Could you check a few things on this model? Use its own coordinates, in mm. Give positions to 0.01 mm unless a question says otherwise; leave off trailing zeros. Loops run counter-clockwise (first coordinate to the right, second up) from the corner with the lowest first, then second, coordinate; pieces in that order, holes last. Notation, with made-up numbers: M -27.75,10.25 L -3.75,10.25 A26 cw -3.75,33.25 Z; hole C 61.25,77.5 d2. An arc over 180 degrees is marked long. Use CSV: the item, a comma, the result in double quotes.
```python
from build123d import *

# Parameters (mm, degrees)
SKETCH1_W             = 5
SKETCH1_H             = 112
BOSS_EXTRUDE1_DEPTH   = 5
SKETCH2_W             = 112
SKETCH2_H             = 5
BOSS_EXTRUDE2_DEPTH   = 145
BOSS_EXTRUDE3_DEPTH   = 107
SKETCH5_W             = 150
SKETCH5_H             = 3
CUT_EXTRUDE1_DEPTH    = 30
CHAMFER1_SIZE         = 2
CHAMFER1_SIZE2        = 1.414213562
CHAMFER1_EDGE_2_SIZE  = 2
CHAMFER1_EDGE_2_SIZE2 = 1.414213562
SKETCH6_W             = 131.302943726
SKETCH6_H             = 15
BOSS_EXTRUDE4_DEPTH   = 2
CUT_EXTRUDE2_DEPTH    = 131.302943725


with BuildPart() as part:
    # Sketch1 → Boss-Extrude1 (new body)
    with BuildSketch(Plane(origin=(0, 0, 0), x_dir=(1, 0, 0), z_dir=(0, 1, 0))):
        Rectangle(SKETCH1_W, SKETCH1_H)
    extrude(amount=BOSS_EXTRUDE1_DEPTH)

    # Sketch2 → Boss-Extrude2 (add)
    with BuildSketch(Plane(origin=(2.5, 0, 0), x_dir=(0, 0, -1), z_dir=(1, 0, 0))):
        with Locations((0, 2.5)):
            Rectangle(SKETCH2_W, SKETCH2_H)
    extrude(amount=BOSS_EXTRUDE2_DEPTH)

    # Sketch3 → Boss-Extrude3 (add)
    with BuildSketch(Plane(origin=(0, 0, -56), x_dir=(-1, 0, 0), z_dir=(0, 0, -1))):
        Polygon((-136.651471863, 0), (-141.251471863, -4.6), (-3.748528137, -4.6), (-8.348528137, 0), align=None)
    extrude(amount=-BOSS_EXTRUDE3_DEPTH)

    # Sketch5 → Cut-Extrude1 (cut)
    with BuildSketch(Plane(origin=(0, 0, -56), x_dir=(-1, 0, 0), z_dir=(0, 0, -1))):
        with Locations((-72.5, 0)):
            Rectangle(SKETCH5_W, SKETCH5_H)
    extrude(amount=-CUT_EXTRUDE1_DEPTH, mode=Mode.SUBTRACT)

    # Chamfer1
    chamfer1_edges = [part.edges().sort_by_distance(p)[0] for p in [
        (3.748528137, -4.6, -2.5),
    ]]
    chamfer1_side = [part.faces().sort_by_distance(p)[0] for p in [
        (72.5, -4.6, -2.5),
    ]]
    chamfer(chamfer1_edges, length=CHAMFER1_SIZE, length2=CHAMFER1_SIZE2, reference=chamfer1_side[0])

    # Chamfer1 edge 2
    chamfer1_edge_2_edges = [part.edges().sort_by_distance(p)[0] for p in [
        (141.251471863, -4.6, -2.5),
    ]]
    chamfer1_edge_2_side = [part.faces().sort_by_distance(p)[0] for p in [
        (72.5, -4.6, -2.5),
    ]]
    chamfer(chamfer1_edge_2_edges, length=CHAMFER1_EDGE_2_SIZE, length2=CHAMFER1_EDGE_2_SIZE2, reference=chamfer1_edge_2_side[0])

    # Sketch6 → Boss-Extrude4 (add)
    with BuildSketch(Plane.XZ.offset(4.6)):
        with Locations((72.5, -43.3)):
            Rectangle(SKETCH6_W, SKETCH6_H)
    extrude(amount=BOSS_EXTRUDE4_DEPTH)

    # Sketch7 → Cut-Extrude2 (cut)
    with BuildSketch(Plane(origin=(138.151471863, 0, 0), x_dir=(0, 0, -1), z_dir=(1, 0, 0))):
        Polygon((35.8, -4.6), (52.8358392, -6.6), (35.8, -6.6), align=None)
    extrude(amount=-CUT_EXTRUDE2_DEPTH, mode=Mode.SUBTRACT)


solid = part.part
```
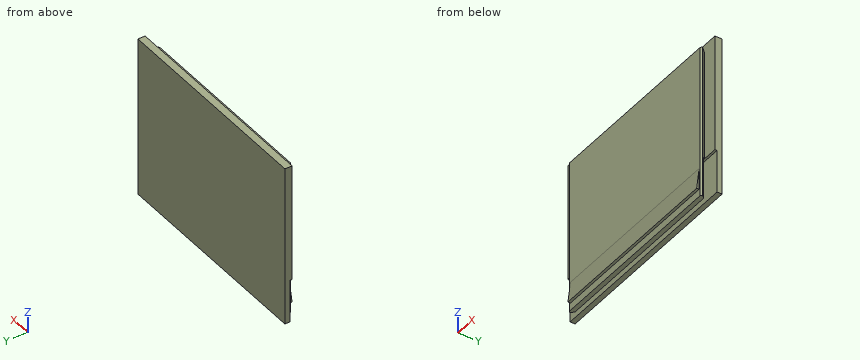
1. I want a section at A-A, the plane z = -32. List the corners of the cut face in (x, y) for me.
Outcome:
outline,"M -2.5,1.5 L 147.5,1.5 L 147.5,5 L -2.5,5 Z; M 4.75,-3.6 L 5.75,-4.6 L 139.25,-4.6 L 140.25,-3.6 L 138.15,-1.5 L 6.85,-1.5 Z"
2. I want a section at D-D, the plane z = -47. List the corners of the cut face in (x, y) for me.
Outcome:
outline,"M -2.5,1.5 L 147.5,1.5 L 147.5,5 L -2.5,5 Z; M 4.75,-3.6 L 5.75,-4.6 L 6.85,-4.6 L 6.85,-5.91 L 138.15,-5.91 L 138.15,-4.6 L 139.25,-4.6 L 140.25,-3.6 L 138.15,-1.5 L 6.85,-1.5 Z"
3. I'm going to push flat-ended pins straight in: pin 1 Ø1.5 at (x, y) = (22, -5) entering from +Z; pin 2 Ø24.5 at (x, z) = (89.5, 8.5) entering from -Y; pin 3 Ø1.9 at (y, z) = (-5.5, -46) entering from -X. Where does each tip first touch, or does it pass through?
Outcome:
pin 1,"z = 51"
pin 2,"y = -4.6"
pin 3,"x = 5.7"
4. Please list where these lines run through material, in increasing order: line 1 (Y direction, x = 122.5, z = -28); line 2 (Z direction, x = 114.5, y = -2); line 3 (Y direction, x = 128.5, z = -42).
Outcome:
line 1,"-4.6 to -1.5, 1.5 to 5"
line 2,"-56 to 51"
line 3,"-5.33 to -1.5, 1.5 to 5"
5. I want a section at C-C, the plane z = -10. List the corners of the cut face in (x, y) for me, then the cut area to 3 significant figures.
Outcome:
outline,"M -2.5,0 L 8.35,0 L 4.75,-3.6 L 5.75,-4.6 L 139.25,-4.6 L 140.25,-3.6 L 136.65,0 L 147.5,0 L 147.5,5 L -2.5,5 Z"
area,"1,360 mm2"
6. I want a section at B-B, the plane x = 28.5. List the corners of the cut face in (y, z) for me, then the cut area to 3 significant figures.
Outcome:
outline,"M -6.36,-50.8 L -4.6,-50.8 L -4.6,-56 L -1.5,-56 L -1.5,-26 L 1.5,-26 L 1.5,-56 L 5,-56 L 5,56 L 0,56 L 0,51 L -4.6,51 L -4.6,-35.8 Z"
area,"975 mm2"
